from build123d import *

# Parameters (mm, degrees)
SKETCH_1_W          = 10
SKETCH_1_H          = 10
EXTRUDE_1_DEPTH     = 10
SKETCH_2_R          = 1.6
CUT_EXTRUDE_1_DEPTH = 10


with BuildPart() as part:
    # Эскиз1 → Бобышка-Вытянуть1 (new body)
    with BuildSketch(Plane.XY):
        with Locations((-25, 4.3)):
            Rectangle(SKETCH_1_W, SKETCH_1_H)
        with BuildLine():
            ThreePointArc((-12.560254774, 9.3), (0, -2.3), (12.560254774, 9.3))
            Line((12.560254774, 9.3), (20, 9.3))
            Line((20, 9.3), (20, -9.3))
            Line((20, -9.3), (-20, -9.3))
            Line((-20, -9.3), (-20, 9.3))
            Line((-20, 9.3), (-12.560254774, 9.3))
        make_face()
        with Locations((25, 4.3)):
            Rectangle(SKETCH_1_W, SKETCH_1_H)
    extrude(amount=EXTRUDE_1_DEPTH)

    # Эскиз2 → Вырез-Вытянуть1 (cut)
    with BuildSketch(Plane(origin=(0, 9.3, 0), x_dir=(1, 0, 0), z_dir=(0, 1, 0))):
        with Locations(Location((25, -5, 0), (0, 0, 270))):
            Circle(SKETCH_2_R)
        with Locations(Location((-25, -5, 0), (0, 0, 90))):
            Circle(SKETCH_2_R)
    extrude(amount=-CUT_EXTRUDE_1_DEPTH, mode=Mode.SUBTRACT)


solid = part.part
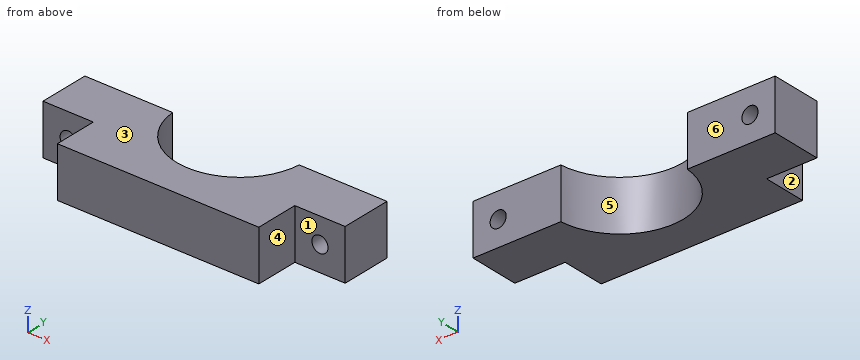
The model under review builds one solid part; all positions refer to its coordinate system, in mm. Face numbers are marked on the shaded views. A direction names the side the tool comes from. Coordinates: 2 decimals unless noted, no trailing zeros. Loops run counter-clockwise (first coordinate to the right, second up) from the corner with the lowest first, then second, coordinate; pieces in that order, holes last. Notation, with made-up numbers: M 76.25,40 L 121.25,40 A22 ccw 121.25,77 Z; hole C 20.25,-2.75 d5. An arc over 180 degrees is marked long. Put each result on its own line as item: value. Start each with the question number.
Q1. Add section A-A (z = 5). Write out the cut boundary in (x, y).
Q2. Clearance check with flat-ended pins moving along their axes: pin 1 (5 mm diameter, centred on x = 26.5, z = 6.5, fed in from -Y); pin 2 (2 mm diameter, centred on y = -3, z = 7, fed in from -X); pin 3 (4.5 mm diameter, centred on y = -6.5, z = 5, fed in from +X). State where each tip first meets the part, or that it passes through.
Q3. Add section C-C (y = 6). Write out the cut boundary in (x, z), and give its area (3 significant figures).
Q4. Add section B-B (x = -25). Write out the cut boundary in (y, z).
Q5. The part is to be moulded in two halves that separate along X. For the marked faces 4, 5 and 6, say which applies: +X half, -X half, draft (parallel to the pull), parting line (faces both ways), or undercut.
Q6. For the marked faces 1, 2 and 3, list the 3-axis set-ups (+Z, -Z, +X, -X, +Y, -Y) from which the entire face can be reached by the end or side of a thin tool; tool diameter is ignored.
Q7. Wall thickness on line 1 (X direction, y = 2.75, z = 5); line 2 (X direction, y = 5.75, z = 5); line 3 (Z direction, x = -25, y = 4): over which ranges is each line inside the solid? List them lowest first.
Q8. Add section D-D (z = 7.5). Write out the cut boundary in (x, y), and give its area (3 significant figures).
Answers:
1. outline: M -30,-0.7 L -26.6,-0.7 L -26.6,9.3 L -30,9.3 Z; M -23.4,-0.7 L -20,-0.7 L -20,-9.3 L 20,-9.3 L 20,-0.7 L 23.4,-0.7 L 23.4,9.3 L 12.56,9.3 A12.6 cw -12.56,9.3 L -23.4,9.3 Z; M 26.6,-0.7 L 30,-0.7 L 30,9.3 L 26.6,9.3 Z
2. pin 1: stops at y = -0.7
2. pin 2: stops at x = -20
2. pin 3: stops at x = 20
3. outline: M -30,0 L -11.84,0 L -11.84,10 L -30,10 Z; M 11.84,0 L 30,0 L 30,10 L 11.84,10 Z; hole C -25,5 d3.2; hole C 25,5 d3.2
3. area: 347 mm^2
4. outline: M -0.7,0 L 9.3,0 L 9.3,3.4 L -0.7,3.4 Z; M -0.7,6.6 L 9.3,6.6 L 9.3,10 L -0.7,10 Z
5. face 4: +X half
5. face 5: undercut
5. face 6: draft
6. face 1: +Z, -Z, +X, -Y
6. face 2: +Z, -Z, -X, -Y
6. face 3: +Z, +X, -X, +Y, -Y
7. line 1: x = -30 to -26.6, -23.4 to -10.09, 10.09 to 23.4, 26.6 to 30
7. line 2: x = -30 to -26.6, -23.4 to -11.75, 11.75 to 23.4, 26.6 to 30
7. line 3: z = 0 to 3.4, 6.6 to 10
8. outline: M -30,-0.7 L -20,-0.7 L -20,-9.3 L 20,-9.3 L 20,-0.7 L 30,-0.7 L 30,9.3 L 12.56,9.3 A12.6 cw -12.56,9.3 L -30,9.3 Z
8. area: 720 mm^2
